Geometry: final body of the model. Coordinates: model frame, mm. Face numbers are marked on the shaded views. Round coordinates to 2 decimals unless told otherwise and drop trailing zeros. Loops run counter-clockwise (first coordinate to the right, second up) from the corner with the lowest first, then second, coordinate; pieces in that order, holes last. Notation, with made-up numbers: (2.25, -18.75) - (29.25, -18.75) arc R10 ccw to (29.25, -8.75) - close; hole circle Ø5 at (5, 60). An arc over 180 degrees is marked (long way). Answer in a Markdown table with one row per item. Add a question column.
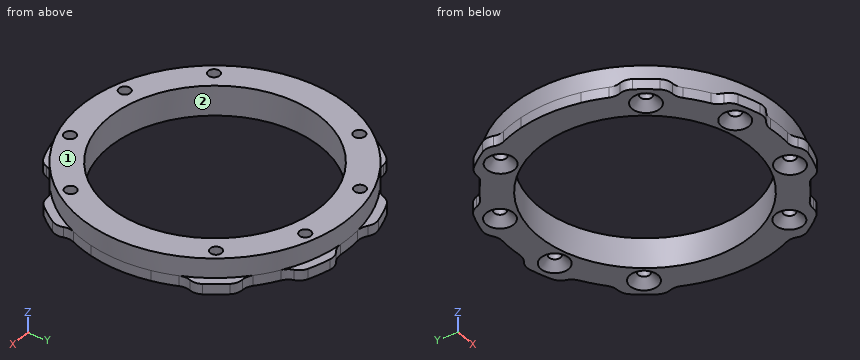
from build123d import *

# Parameters (mm, degrees)
SKIZZE1_R                       = 18.5
LINEAR_AUSTRAGEN1_DEPTH         = 1.8
SKIZZE2_R                       = 23.4
SKIZZE2_R_2                     = 18.5
LINEAR_AUSTRAGEN2_DEPTH         = 3.4
SKIZZE3_R                       = 1
SCHNITT_LINEAR_AUSTRAGEN1_DEPTH = 35.115425177
CHAMFER1_SIZE                   = 1.4


with BuildPart() as part:
    # Skizze1 → Linear austragen1 (new body)
    with BuildSketch(Plane.XY):
        with BuildLine():
            ThreePointArc((-22.806936421, 5.234849671), (-23.4, 0), (-22.806936421, -5.234849671))
            ThreePointArc((-22.806936421, -5.234849671), (-22.254722481, -7.230997668), (-21.528166589, -9.170498531))
            ThreePointArc((-21.528166589, -9.170498531), (-21.322328126, -10.083900652), (-21.453393631, -11.010990043))
            ThreePointArc((-21.453393631, -11.010990043), (-21.560643818, -12.043510102), (-21.221833257, -13.024737741))
            ThreePointArc((-21.221833257, -13.024737741), (-20.14452316, -14.635852782), (-18.94516883, -16.158297497))
            ThreePointArc((-18.94516883, -16.158297497), (-18.116664111, -16.783741505), (-17.10153705, -17.000806761))
            ThreePointArc((-17.10153705, -17.000806761), (-16.179321175, -17.162642436), (-15.37423172, -17.640663225))
            ThreePointArc((-15.37423172, -17.640663225), (-13.754174904, -18.930997668), (-12.026368835, -20.073027989))
            ThreePointArc((-12.026368835, -20.073027989), (-11.322957725, -20.690997014), (-10.884062474, -21.518066457))
            ThreePointArc((-10.884062474, -21.518066457), (-10.363929634, -22.416432811), (-9.513074997, -23.011114795))
            ThreePointArc((-9.513074997, -23.011114795), (-7.69452316, -23.681307256), (-5.829354574, -24.208028116))
            ThreePointArc((-5.829354574, -24.208028116), (-4.791453413, -24.227040092), (-3.842610612, -23.805972857))
            ThreePointArc((-3.842610612, -23.805972857), (-3.001397674, -23.394835778), (-2.069093052, -23.308343012))
            ThreePointArc((-2.069093052, -23.308343012), (0, -23.4), (2.069093052, -23.308343012))
            ThreePointArc((2.069093052, -23.308343012), (3.001397674, -23.394835778), (3.842610612, -23.805972857))
            ThreePointArc((3.842610612, -23.805972857), (4.791453413, -24.227040092), (5.829354574, -24.208028116))
            ThreePointArc((5.829354574, -24.208028116), (7.69452316, -23.681307256), (9.513074997, -23.011114795))
            ThreePointArc((9.513074997, -23.011114795), (10.363929634, -22.416432811), (10.884062474, -21.518066457))
            ThreePointArc((10.884062474, -21.518066457), (11.322957725, -20.690997014), (12.026368835, -20.073027989))
            ThreePointArc((12.026368835, -20.073027989), (13.754174904, -18.930997668), (15.37423172, -17.640663225))
            ThreePointArc((15.37423172, -17.640663225), (16.179321175, -17.162642436), (17.10153705, -17.000806761))
            ThreePointArc((17.10153705, -17.000806761), (18.116664111, -16.783741505), (18.94516883, -16.158297497))
            ThreePointArc((18.94516883, -16.158297497), (20.14452316, -14.635852782), (21.221833257, -13.024737741))
            ThreePointArc((21.221833257, -13.024737741), (21.560643818, -12.043510102), (21.453393631, -11.010990043))
            ThreePointArc((21.453393631, -11.010990043), (21.322328126, -10.083900652), (21.528166589, -9.170498531))
            ThreePointArc((21.528166589, -9.170498531), (22.254722481, -7.230997668), (22.806936421, -5.234849671))
            ThreePointArc((22.806936421, -5.234849671), (23.4, 0), (22.806936421, 5.234849671))
            ThreePointArc((22.806936421, 5.234849671), (22.254722481, 7.230997668), (21.528166589, 9.170498531))
            ThreePointArc((21.528166589, 9.170498531), (21.322328126, 10.083900652), (21.453393631, 11.010990043))
            ThreePointArc((21.453393631, 11.010990043), (21.560643818, 12.043510102), (21.221833257, 13.024737741))
            ThreePointArc((21.221833257, 13.024737741), (20.14452316, 14.635852782), (18.94516883, 16.158297497))
            ThreePointArc((18.94516883, 16.158297497), (18.116664111, 16.783741505), (17.10153705, 17.000806761))
            ThreePointArc((17.10153705, 17.000806761), (16.179321175, 17.162642436), (15.37423172, 17.640663225))
            ThreePointArc((15.37423172, 17.640663225), (13.754174904, 18.930997668), (12.026368835, 20.073027989))
            ThreePointArc((12.026368835, 20.073027989), (11.322957725, 20.690997014), (10.884062474, 21.518066457))
            ThreePointArc((10.884062474, 21.518066457), (10.363929634, 22.416432811), (9.513074997, 23.011114795))
            ThreePointArc((9.513074997, 23.011114795), (7.69452316, 23.681307256), (5.829354574, 24.208028116))
            ThreePointArc((5.829354574, 24.208028116), (4.791453413, 24.227040092), (3.842610612, 23.805972857))
            ThreePointArc((3.842610612, 23.805972857), (3.001397674, 23.394835778), (2.069093052, 23.308343012))
            ThreePointArc((2.069093052, 23.308343012), (0, 23.4), (-2.069093052, 23.308343012))
            ThreePointArc((-2.069093052, 23.308343012), (-3.001397674, 23.394835778), (-3.842610612, 23.805972857))
            ThreePointArc((-3.842610612, 23.805972857), (-4.791453413, 24.227040092), (-5.829354574, 24.208028116))
            ThreePointArc((-5.829354574, 24.208028116), (-7.69452316, 23.681307256), (-9.513074997, 23.011114795))
            ThreePointArc((-9.513074997, 23.011114795), (-10.363929634, 22.416432811), (-10.884062474, 21.518066457))
            ThreePointArc((-10.884062474, 21.518066457), (-11.322957725, 20.690997014), (-12.026368835, 20.073027989))
            ThreePointArc((-12.026368835, 20.073027989), (-13.754174904, 18.930997668), (-15.37423172, 17.640663225))
            ThreePointArc((-15.37423172, 17.640663225), (-16.179321175, 17.162642436), (-17.10153705, 17.000806761))
            ThreePointArc((-17.10153705, 17.000806761), (-18.116664111, 16.783741505), (-18.94516883, 16.158297497))
            ThreePointArc((-18.94516883, 16.158297497), (-20.14452316, 14.635852782), (-21.221833257, 13.024737741))
            ThreePointArc((-21.221833257, 13.024737741), (-21.560643818, 12.043510102), (-21.453393631, 11.010990043))
            ThreePointArc((-21.453393631, 11.010990043), (-21.322328126, 10.083900652), (-21.528166589, 9.170498531))
            ThreePointArc((-21.528166589, 9.170498531), (-22.254722481, 7.230997668), (-22.806936421, 5.234849671))
        make_face()
        Circle(SKIZZE1_R, mode=Mode.SUBTRACT)
    extrude(amount=LINEAR_AUSTRAGEN1_DEPTH)

    # Skizze2 → Linear austragen2 (add)
    with BuildSketch(Plane.XY.offset(1.8)):
        with Locations(Location((0, 0, 0), (0, 0, 156.927122734))):
            Circle(SKIZZE2_R)
        Circle(SKIZZE2_R_2, mode=Mode.SUBTRACT)
    extrude(amount=LINEAR_AUSTRAGEN2_DEPTH)

    # Skizze3 → Schnitt-Linear austragen1 (cut, through all)
    with BuildSketch(Plane.XY.offset(5.2)):
        with Locations((-6.643865379, 20.4477151)):
            Circle(SKIZZE3_R)
        with Locations((6.643865379, 20.4477151)):
            Circle(SKIZZE3_R)
        with Locations((17.393865379, 12.637382924)):
            Circle(SKIZZE3_R)
        with Locations((17.393865379, -12.637382924)):
            Circle(SKIZZE3_R)
        with Locations((6.643865379, -20.4477151)):
            Circle(SKIZZE3_R)
        with Locations((-6.643865379, -20.4477151)):
            Circle(SKIZZE3_R)
        with Locations((-17.393865379, -12.637382924)):
            Circle(SKIZZE3_R)
        with Locations((-17.393865379, 12.637382924)):
            Circle(SKIZZE3_R)
    extrude(amount=-SCHNITT_LINEAR_AUSTRAGEN1_DEPTH, mode=Mode.SUBTRACT)

    # Chamfer1
    chamfer1_edges = [part.edges().sort_by_distance(p)[0] for p in [
        (-7.643865379, 20.4477151, 0),
        (5.643865379, 20.4477151, 0),
        (16.393865379, 12.637382924, 0),
        (16.393865379, -12.637382924, 0),
        (5.643865379, -20.4477151, 0),
        (-7.643865379, -20.4477151, 0),
        (-18.393865379, -12.637382924, 0),
        (-18.393865379, 12.637382924, 0),
    ]]
    chamfer(chamfer1_edges, length=CHAMFER1_SIZE)


solid = part.part
1) Section A-A, the plane x = 0. Return the cut outline in (y, z).
2) Contact query for a flat-ended pin moving along its axis: pin 1 Ø3 at (x, y) = (6.64, 20.45) entering from -Z. Output: stop coordinate, or through.
3) Material intervals for line 1 along X through (y, z) = (-20, 1.45); line 2 along X through (y, z) = (12.5, 4.9); line 3 along X through (y, z) = (-17, 3.3), sorted ascending. Write a range as from..to.
4) Section D-D, the plane x = 13. Return the cut outline in (y, z), and give its area (3 significant figures).
5) Pull-direction query (Y, two-part tool) for the marked faces 1 and 2; classes: pulls with the +Y half, pulls with the -Y half, needs draft (parallel to the pull), parting line crosses it, or undercut.
6) Section C-C, the plane z = 2.4. Give the number of separate pieces and of enclosed holes in the cut face, and give its area (3 significant figures).
Evaluation:
| question | item | result |
|---|---|---|
| 1 | outline | (-23.4, 0) - (-18.5, 0) - (-18.5, 5.2) - (-23.4, 5.2) - close; (18.5, 0) - (23.4, 0) - (23.4, 5.2) - (18.5, 5.2) - close |
| 2 | pin 1 | stops at z = 0.9 |
| 3 | line 1 | x = -12.15..-7.54, -5.75..5.75, 7.54..12.15 |
| 3 | line 2 | x = -19.78..-18.38, -16.4..-13.64, 13.64..16.4, 18.38..19.78 |
| 3 | line 3 | x = -16.08..-7.3, 7.3..16.08 |
| 4 | outline | (-19.46, 0) - (-13.16, 0) - (-13.16, 5.2) - (-19.46, 5.2) - close; (13.16, 0) - (19.46, 0) - (19.46, 5.2) - (13.16, 5.2) - close |
| 4 | area | 65.5 mm² |
| 5 | face 1 | needs draft |
| 5 | face 2 | undercut |
| 6 | separate pieces | 1 |
| 6 | enclosed holes | 9 |
| 6 | area | 620 mm² |
